For this review, take the finished solid that the model builds, in its own axes (mm). Face numbers are marked on the shaded views. A direction names the side the tool comes from. Coordinates: 2 decimals unless noted, no trailing zeros. Order: outer loops, then holes, each group sorted by start corner. A loop starts at its lowest first (then second) coordinate and runs counter-clockwise, first axis right, second up. Notation, with made-up numbers: (-23.5, -22) - (7.5, -22) arc R30 cw to (7.5, 7) - close; hole circle Ø2 at (32, 87.5). An arc over 180 degrees is marked (long way). One line per item, written item: value. Start each with the question number.
(1) For the marked faces 1, 2, 3, 4 and 5, list the 3-axis set-ups (+Z, -Z, +X, -X, +Y, -Y) from which the entire face can be reached by the end or side of a thin tool; tool diameter is ignored.
(2) Consider section D-D on z = -9. Write out the cut boundary in (x, y), then the cut area to 3 significant figures.
(3) Consider section A-A on y = -21.75. Write out the cut boundary in (x, z), then the cut area to 3 significant figures.
(4) Clearance check with flat-ended pins moving along their axes: pin 1 (2.5 mm diameter, centred on y = -27.5, z = 5.5, fed in from +X); pin 2 (4 mm diameter, centred on x = 1, y = -28.5, fed in from -Z); pin 3 (3 mm diameter, centred on y = -25, z = -9, fed in from -X). State where each tip first meets the part, or that it passes through.
(5) Consider section C-C on z = 0. Write out the cut boundary in (x, y).
(6) Mouldability with a two-part tool opening along Y and no side actions: class the marked faces 6, 7, 8 and 9 as released by +Y, released by -Y, zero draft, split by the parting line, or undercut.
(7) To check wall thickness, follow line 1 along X through (y, z) = (-26.25, 7.25); line 2 along Y through (x, z) = (5.5, -2.5); line 3 along X through (y, z) = (-10, 7.75). State the ranges of each line that lie inside material, in increasing order.
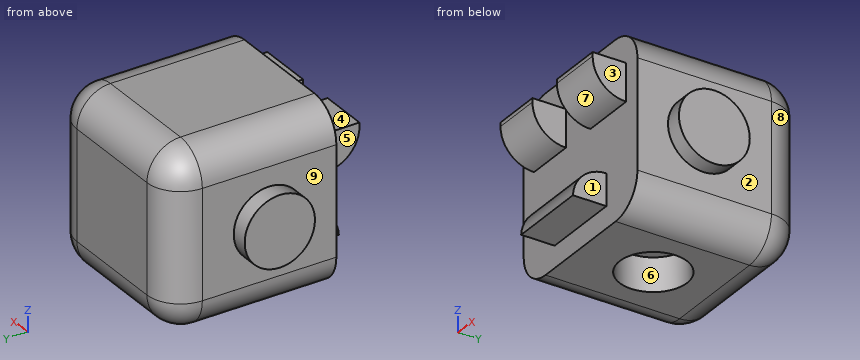
```python
from build123d import *

# Parameters (mm, degrees)
F0_W        = 25.9993169457
F0_H        = 26.2141898274
F1_DEPTH    = 25
F2_R        = 5
F3_W        = 8.165073581
F3_H        = 5.5866301991
F3_W_2      = 7.3055946268
F4_W        = 11.8178697303
F4_H        = 4.7271503136
F5_DEPTH    = 5
F6_T1_DEPTH = 32.3055946268
F6_T3_DEPTH = 33.165073581
F6_T5_DEPTH = 36.7806185015
F7_R        = 5.2851135751
F9_DEPTH    = 2.5
F8_R        = 5.2456555176
F10_DEPTH   = 2.5
F11_R       = 5.0288488875
F12_DEPTH   = 5


# Not quite as in the source:
# - a fillet or chamfer that OpenCascade refuses, or shapes differently, is made with other operations: its cross-section is extruded or revolved along the edge and cut away or added


with BuildPart() as f1:
    # F0 (on Front) → F1 (new body)
    with BuildSketch(Plane.XZ):
        Rectangle(F0_W, F0_H)
    extrude(amount=F1_DEPTH)

    # F2
    f2_edges = [f1.edges().sort_by_distance(p)[0] for p in [
        (-12.999658, -12.5, 13.107095),
        (0, 0, 13.107095),
        (12.999658, -12.5, 13.107095),
        (12.999658, 0, 0),
        (12.999658, -12.5, -13.107095),
        (-12.999658, -12.5, -13.107095),
        (0, 0, -13.107095),
        (-12.999658, 0, 0),
    ]]
    fillet(f2_edges, radius=F2_R)

    # F3 (on face) + F4 (on face) → F5 (join)
    with BuildSketch(Plane.XZ.offset(25)):
        with Locations((6.3386769034, 5.8015007526)):
            Rectangle(F3_W, F3_H)
        with Locations((-6.9832885638, 5.8015007526)):
            Rectangle(F3_W_2, F3_H)
    with BuildSketch(Plane.XZ.offset(25)):
        with Locations((0, -7.5204637833)):
            Rectangle(F4_W, F4_H)
    extrude(amount=F5_DEPTH)

    # F6: fillet of radius 5 on 3 edges, made by hand

    # F6_s2 → F6_t1 (cut)
    with BuildSketch(Plane.YZ.offset(-23.1360858772)):
        with BuildLine():
            ThreePointArc((-25, 3.008185653), (-28.5355339059, 4.4726517471), (-30, 8.008185653))
            Line((-30, 8.008185653), (-30, 3.008185653))
            Line((-30, 3.008185653), (-25, 3.008185653))
        make_face()
    extrude(amount=F6_T1_DEPTH, mode=Mode.SUBTRACT)

    # F6_s4 → F6_t3 (cut)
    with BuildSketch(Plane.YZ.offset(-10.2438598871)):
        with BuildLine():
            ThreePointArc((-25, 3.008185653), (-28.5355339059, 4.4726517471), (-30, 8.008185653))
            Line((-30, 8.008185653), (-30, 3.008185653))
            Line((-30, 3.008185653), (-25, 3.008185653))
        make_face()
    extrude(amount=F6_T3_DEPTH, mode=Mode.SUBTRACT)

    # F6_s6 → F6_t5 (cut)
    with BuildSketch(Plane.YZ.offset(-18.3903092508)):
        with BuildLine():
            ThreePointArc((-25.0074502458, -5.1568886265), (-28.4451639895, -6.5261691088), (-30, -9.8840389401))
            Line((-30, -9.8840389401), (-30, -5.1568886265))
            Line((-30, -5.1568886265), (-25.0074502458, -5.1568886265))
        make_face()
    extrude(amount=F6_T5_DEPTH, mode=Mode.SUBTRACT)

    # F7 (on face) → F9 (join)
    with BuildSketch(Plane.YZ.offset(12.9996584728)):
        with Locations((-15.1483640075, 0)):
            Circle(F7_R)
    extrude(amount=F9_DEPTH)

    # F8 (on face) → F10 (join)
    with BuildSketch(Plane(origin=(-12.9996584728, 0, 0), x_dir=(0, -1, 0), z_dir=(-1, 0, 0))):
        with Locations((14.9334929883, 0)):
            Circle(F8_R)
    extrude(amount=F10_DEPTH)

    # F11 (on face) → F12 (cut)
    with BuildSketch(Plane(origin=(0, 0, -13.1070949137), x_dir=(1, 0, 0), z_dir=(0, 0, -1))):
        with Locations((0, 14.1341807321)):
            Circle(F11_R)
    extrude(amount=-F12_DEPTH, mode=Mode.SUBTRACT)


solid = f1.part
```
Geometry check:
1. face 1: -Z, +X, -Y
1. face 2: +X
1. face 3: +Z, -Z, +X, -Y
1. face 4: +Z, +X, -X, -Y
1. face 5: +Z, -Z, -X, -Y
2. outline: (-12.92, -25) - (-5.91, -25) - (-5.91, -29.87) - (5.91, -29.87) - (5.91, -25) - (12.92, -25) - (12.92, -5) arc R4.92 ccw to (8, -0.08) - (-8, -0.08) arc R4.92 ccw to (-12.92, -5) - close; hole circle Ø10.06 at (0, -14.13)
2. area: 612 mm^2
3. outline: (-13, -8.11) arc R5 ccw to (-8, -13.11) - (8, -13.11) arc R5 ccw to (13, -8.11) - (13, 8.11) arc R5 ccw to (8, 13.11) - (-8, 13.11) arc R5 ccw to (-13, 8.11) - close
3. area: 660 mm^2
4. pin 1: stops at x = 10.42
4. pin 2: stops at z = -9.88
4. pin 3: stops at x = -13
5. outline: (-15.5, -20.18) - (-13, -20.18) - (-13, -25) - (13, -25) - (13, -20.43) - (15.5, -20.43) - (15.5, -9.86) - (13, -9.86) - (13, -5) arc R5 ccw to (8, 0) - (-8, 0) arc R5 ccw to (-13, -5) - (-13, -9.69) - (-15.5, -9.69) - close
6. face 6: undercut
6. face 7: released by -Y
6. face 8: released by +Y
6. face 9: zero draft
7. line 1: x = -10.64 to -3.33, 2.26 to 10.42
7. line 2: y = -25 to 0
7. line 3: x = -13 to 13
